Check sheet for the modelled part. Datum: model origin and axes. Units: mm. A direction names the side the tool comes from. Give positions to 0.01 mm unless a question says otherwise; leave off trailing zeros. Write each loop counter-clockwise with the first axis right and the second up, starting at its lowest first coordinate (ties: lowest second). Pieces come first, ordered by that corner, then holes. Notation, with made-up numbers: (30.5, 10) -> (53.5, 10) arc R14 ccw to (53.5, 32) -> close; hole circle Ø7 at (-16, 74.5). An arc over 180 degrees is marked (long way). Return JSON: item names as keys, results as strings.
Autodesk Inventor part; units mm, degrees
ref_plane "YZ Plane" through (0, 0, 0) normal (1, 0, 0) x (0, 1, 0)
ref_plane "XZ Plane" through (0, 0, 0) normal (0, 1, 0) x (-1, 0, 0)
ref_plane "XY Plane" through (0, 0, 0) normal (0, 0, 1) x (1, 0, 0)
sketch "Sketch1" plane through (0, 0, 0) normal (0, 0, 1) x (1, 0, 0)
  circle A0 centre (7.161, 8.0403) radius 1.524
  line L0 (16.461, -12.7743) -> (16.461, -7.3635)
  arc A1 (16.461, -7.3635) -> (16.2925, -6.0336) centre (11.127, -7.3635) ccw
  line L1 (16.2925, -6.0336) -> (12.3265, 9.3703)
  arc A2 (12.3265, 9.3703) -> (7.161, 13.3743) centre (7.161, 8.0403) ccw
  line L2 (7.161, 13.3743) -> (-11.127, 13.3743)
  arc A3 (-11.127, 13.3743) -> (-16.461, 8.0403) centre (-11.127, 8.0403) ccw
  line L3 (-16.461, 8.0403) -> (-16.461, -8.0403)
  arc A4 (-16.461, -8.0403) -> (-11.127, -13.3743) centre (-11.127, -8.0403) ccw
  line L4 (-11.127, -13.3743) -> (15.861, -13.3743)
  arc A5 (15.861, -13.3743) -> (16.461, -12.7743) centre (15.861, -12.7743) ccw
  circle A6 centre (-11.127, 8.0403) radius 4.064
  circle A7 centre (7.161, 8.0403) radius 1.6002
  circle A8 centre (7.161, 8.0403) radius 2.032
  circle A9 centre (7.161, 8.0403) radius 1.905
  point P0 (0, 0)
  dimension "d0" = 0.0762
  dimension "d1" = 0.127
extrude "Extrusion1" add sketch "Sketch1" along normal blind 2.3495 contours A9
fillet "Fillet1" radius 0.127 2 edges at (5.5608, 8.0403, 2.3495) (5.5608, 8.0403, 0)
sketch "Sketch2" plane through (7.161, 8.0403, 0) normal (0, 0, -1) x (-1, 0, 0)
  circle A0 centre (0, 0) radius 1.905
  circle A1 centre (0, 0) radius 3.175
  point P0 (7.161, -8.0403)
  dimension "d5" = 6.35
extrude "Extrusion2" add sketch "Sketch2" against normal blind 0.381
properties part number "M3Spacer"
(1) Depth check by flat-ended pin: pin 1 Ø1 at (x, z) = (8, 1) entering from -Y; pin 2 Ø1 at (y, z) = (6.5, 1) entering from -X. Enter the tip coordinate at first touch or a pass-through.
Reply:
{"pin 1": "y = 6.17", "pin 2": "x = 5.57"}
(2) Thickness scan on L1, parallel to Y at x = 7.25, z = 0.25; L2, parallel to X at y = 8, z = 2.2; L3, parallel to X at y = 9.25, z = 1.75. Record the ranges inside material, lowest first.
Reply:
{"L1": "4.87 to 6.44, 9.64 to 11.21", "L2": "5.26 to 5.56, 8.76 to 9.07", "L3": "5.69 to 6.11, 8.21 to 8.63"}
(3) Release check for a two-part mould opening along X. For faces 3 (the cylindrical face through (8.185, 6.434, 1.351)), 4 (the flat face through (5.8, 6.7, 0)), 5 (the cylindrical face through (5.98, 6.96, 1.16)) record: pulls with the +X half, pulls with the -X half, needs draft (parallel to the pull), parting line crosses it, or undercut.
Reply:
{"face 3": "parting line crosses it", "face 4": "needs draft", "face 5": "undercut"}
(4) Set-up check for faces 1 (the flat face through (5, 8, 0.381)), 2 (the cylindrical face through (7.85, 4.94, 0.19)): record each of +Z, -Z, +X, -X, +Y, -Y from which the full face is reachable in a straight line by a thin tool's end or side.
Reply:
{"face 1": "+Z", "face 2": "+Z, -Z"}
(5) Cross-section at B-B on x = 9.5. Enter the section's corners in (y, z), then the cut area to 3 significant figures.
Reply:
{"outline": "(5.89, 0) -> (10.19, 0) -> (10.19, 0.38) -> (5.89, 0.38) -> close", "area": "1.64 mm^2"}
(6) Cross-section at C-C on x = 5. Enter the section's corners in (y, z).
Reply:
{"outline": "(5.71, 0) -> (10.37, 0) -> (10.37, 0.38) -> (5.71, 0.38) -> close"}
(7) Cross-section at A-A on z = 0.7. Enter the section's corners in (x, y) (3 decimals).
Reply:
{"outline": "circle Ø3.81 at (7.161, 8.04); hole circle Ø3.2 at (7.161, 8.04)"}
